from build123d import *

# Parameters (mm, degrees)
F0_W     = 72
F0_H     = 2
F1_DEPTH = 2
F2_DEPTH = 30
F3_W     = 23.2293857262
F3_H     = 26.1833476555
F4_DEPTH = 2
F5_R     = 0.99999


# Not quite as in the source:
# - a fillet or chamfer is up to 0.001 mm smaller than in the source, because OpenCascade refuses the exact size


with BuildPart() as f1:
    # F0 (on Top) → F1 (new body)
    with BuildSketch(Plane.XY):
        with BuildLine():
            ThreePointArc((-36, 15.5704873412), (0, 22), (36, 15.5704873412))
            Line((36, 15.5704873412), (36, 17.6995486449))
            ThreePointArc((36, 17.6995486449), (0, 24), (-36, 17.6995486449))
            Line((-36, 17.6995486449), (-36, 15.5704873412))
        make_face()
        with BuildLine():
            Line((-40, 14), (40, 14))
            ThreePointArc((40, 14), (38.0081123923, 14.8059057722), (36, 15.5704873412))
            ThreePointArc((36, 15.5704873412), (0, 22), (-36, 15.5704873412))
            ThreePointArc((-36, 15.5704873412), (-38.0081123923, 14.8059057722), (-40, 14))
        make_face()
        Polygon((36, -14), (40, -14), (40, 14), (-40, 14), (-40, -14), (-36, -14), align=None)
        with Locations((0, -15)):
            Rectangle(F0_W, F0_H)
        with BuildLine():
            ThreePointArc((-36, 17.6995486449), (0, 24), (36, 17.6995486449))
            ThreePointArc((36, 17.6995486449), (39.0180800363, 16.5575437512), (42, 15.3242004848))
            Line((42, 15.3242004848), (42, 37))
            Line((42, 37), (-42, 37))
            Line((-42, 37), (-42, 15.3242004848))
            ThreePointArc((-42, 15.3242004848), (-39.0180800363, 16.5575437512), (-36, 17.6995486449))
        make_face()
        Polygon((42, -16), (36, -16), (-36, -16), (-42, -16), (-42, -23), (42, -23), align=None)
    extrude(amount=F1_DEPTH)

    # F0 (on Top) → F2 (join)
    with BuildSketch(Plane.XY):
        with BuildLine():
            Line((-36, -16), (-36, -14))
            Line((-36, -14), (-40, -14))
            Line((-40, -14), (-40, 14))
            ThreePointArc((-40, 14), (-38.0081123923, 14.8059057722), (-36, 15.5704873412))
            Line((-36, 15.5704873412), (-36, 17.6995486449))
            ThreePointArc((-36, 17.6995486449), (-39.0180800363, 16.5575437512), (-42, 15.3242004848))
            Line((-42, 15.3242004848), (-42, -16))
            Line((-42, -16), (-36, -16))
        make_face()
        with BuildLine():
            Line((40, 14), (40, -14))
            Line((40, -14), (36, -14))
            Line((36, -14), (36, -16))
            Line((36, -16), (42, -16))
            Line((42, -16), (42, 15.3242004848))
            ThreePointArc((42, 15.3242004848), (39.0180800363, 16.5575437512), (36, 17.6995486449))
            Line((36, 17.6995486449), (36, 15.5704873412))
            ThreePointArc((36, 15.5704873412), (38.0081123923, 14.8059057722), (40, 14))
        make_face()
    extrude(amount=F2_DEPTH)

    # F3 (on face) → F4 (cut, through all)
    with BuildSketch(Plane(origin=(-42, 0, 0), x_dir=(0, -1, 0), z_dir=(-1, 0, 0))):
        with Locations((0.0190031715, 16.9083261723)):
            Rectangle(F3_W, F3_H)
    extrude(amount=-F4_DEPTH, mode=Mode.SUBTRACT)

    # F5 (radius 1 in the source; OpenCascade refuses exactly that, so slightly less here)
    f5_edges = [f1.edges().sort_by_distance(p)[0] for p in [
        (0, -23, 2),
        (42, -23, 1),
        (42, -19.5, 2),
        (-42, -19.5, 2),
        (-42, 26.1621, 2),
        (0, 37, 2),
        (-42, 37, 1),
        (42, 26.1621, 2),
        (42, 37, 1),
        (42, 15.3242, 16),
        (42, -16, 16),
        (36, 17.699549, 16),
        (36, 15.570487, 16),
        (36, -16, 16),
        (36, -14, 16),
        (-42, 15.3242, 16),
        (-36, 17.699549, 16),
        (-42, 11.59569, 16.908326),
        (-42, -11.633696, 16.908326),
        (-42, -16, 16),
        (-36, -16, 16),
        (-36, -14, 16),
        (-36, 15.570487, 16),
        (-40, -11.633696, 16.908326),
        (-40, 11.59569, 16.908326),
        (-42, -0.019003, 3.816652),
        (-40, -0.019003, 3.816652),
        (-41, -11.633696, 3.816652),
        (-41, 11.59569, 3.816652),
    ]]
    fillet(f5_edges, radius=F5_R)


solid = f1.part
CAD build for the part. Positions are in the model's coordinates, mm. A direction names the side the tool comes from. Coordinates: 2 decimals unless noted, no trailing zeros. Write each loop counter-clockwise with the first axis right and the second up, starting at its lowest first coordinate (ties: lowest second). Pieces come first, ordered by that corner, then holes. Notation, with made-up numbers: M 35,40.25 L 53,40.25 A23 cw 53,78.25 Z; hole C 22.5,54 d11. An arc over 180 degrees is marked long. Answer as a JSON object with one key per item and string values. Group by question number.
1) Mould opens along X. For faces 4 (the face through (39, -14, 16)), 5 (the face through (-39.351, 16.425, 15.764)), 6 (the face through (39.41, 16.4, 15.76)), 7 (the face through (-38.35, 14.67, 15.8)) say: +X half, -X half, draft (parallel to the pull), parting line (faces both ways), or undercut.
2) Pin check, flat tips, straight feed: pin 1 Ø3 at (x, z) = (39.5, 10.5) entering from -Y; pin 2 Ø3 at (x, y) = (26, -4) entering from -Z; pin 3 Ø0.9 at (x, z) = (39, 12.5) entering from +Y; pin 4 Ø14 at (y, z) = (1, 12) entering from -X. Stop position of each tip, or through.
3) Wall check: line 1 (X direction, y = -13, z = 27.5); line 2 (Z direction, x = 17, y = -12); line 3 (X direction, y = 3, z = 19.5). Give the ranges that are in metal, low to high. Write a range as from..to.
4) Tool access for faces 1 (the face through (39, -16, 16)), 2 (the face through (42, 0, 15)), 3 (the face through (38.306, 14.688, 15.804)): list every direction of +Z, -Z, +X, -X, +Y, -Y with a clear straight run to the whole face (end or side of a thin tool).
5) Saw through at B-B (x = 8). Write the cut outline in (y, z).
6) Saw through at D-D (y = 22). Write the cut outline in (x, z).
7) Saw through at C-C (z = 28). Give the number of separate pieces and of enclosed holes in the cut face, plus the area to 3 significant figures.
Values follow:
{
 "1": {"face 4": "undercut", "face 5": "-X half", "face 6": "+X half", "face 7": "undercut"},
 "2": {"pin 1": "stops at y = -16", "pin 2": "stops at z = 0", "pin 3": "stops at y = 16.74", "pin 4": "stops at x = 40"},
 "3": {"line 1": "x = -42..-40, 40..42", "line 2": "z = 0..2", "line 3": "x = 40..42"},
 "4": {"face 1": "+Z, +X, -X, -Y", "face 2": "+Z, -Z, +X, +Y, -Y", "face 3": "+Z"},
 "5": {"outline": "M -23,0 L 37,0 L 37,1 A1 ccw 36,2 L -22,2 A1 ccw -23,1 Z"},
 "6": {"outline": "M -42,0 L 42,0 L 42,1 A1 ccw 41,2 L -41,2 A1 ccw -42,1 Z"},
 "7": {"separate pieces": "3", "enclosed holes": "0", "area": "110 mm2"}
}
